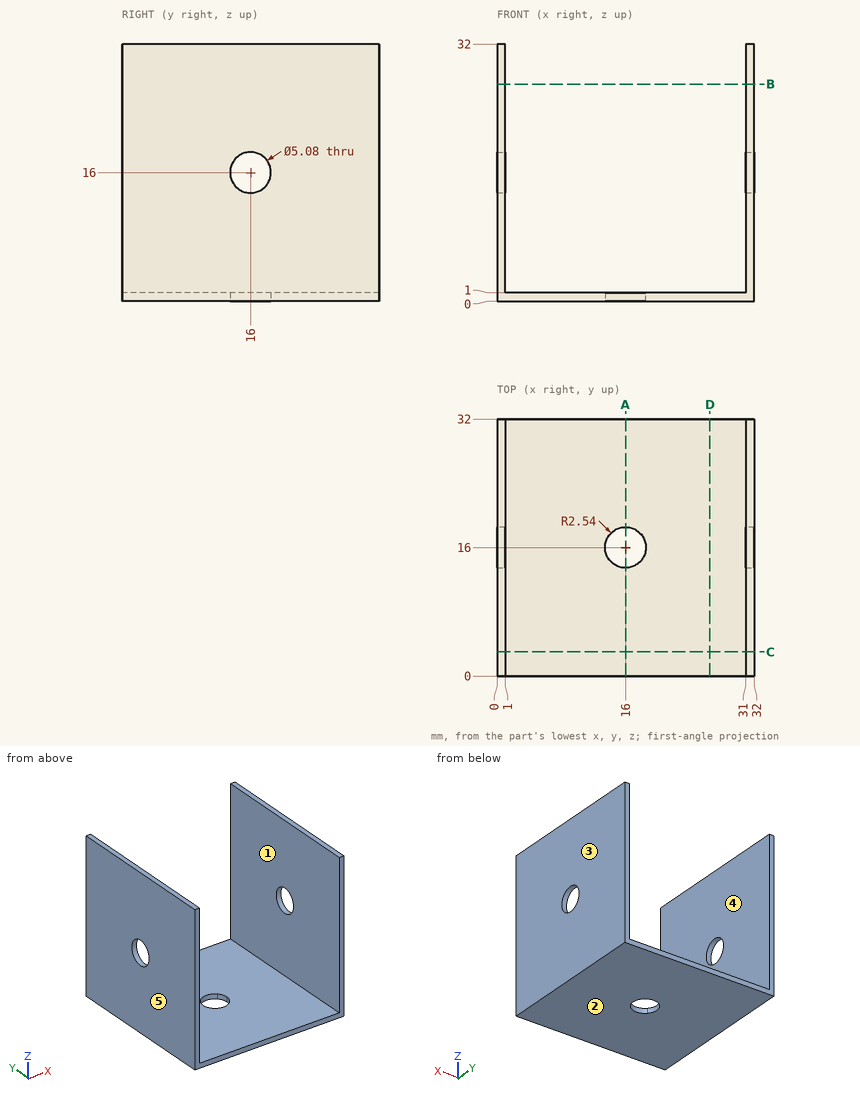
Here's the drawing with two shaded views (mm, measured from the low corner). I have some questions. A direction names the side the tool comes from. Give positions to 0.01 mm unless a question says otherwise; leave off trailing zeros. Loops run counter-clockwise (first coordinate to the right, second up) from the corner with the lowest first, then second, coordinate; pieces in that order, holes last. Notation, with made-up numbers: (-19.5, 84.25) - (-11.5, 84.25) arc R23 ccw to (-11.5, 117.25) - close; hole circle Ø4 at (81, 73). An arc over 180 degrees is marked (long way). Answer in a Markdown table with one row per item. Add a question column.
Q1. If we section it at D-D (x = 26.5): List the corners of the cut face in (y, z) for me.
Q2. For pin 1 (4.5 mm diameter, centred on y = 16, z = 16, fed in from +X); pin 2 (4 mm diameter, centred on x = 25.5, y = 4.5, fed in from +Z), each with a flat end and sliding along its axis, tell me the tip position at first contact or that it passes through.
Q3. We'd pull the mould along X, two halves only. Please class the marked faces 3, 4 and 5: +X half, -X half, draft (parallel to the pull), parting line (faces both ways), or undercut.
Q4. Which directions (+Z, -Z, +X, -X, +Y, -Y) give clear straight access to the entire face, cutting with the end or side of a thin tool? Please do the marked faces 1 and 2.
Q5. If we section it at B-B (z = 27): List the corners of the cut face in (x, y) for me, plus the area to 3 significant figures.
Q6. If we section it at A-A (x = 16): List the corners of the cut face in (y, z) for me.
Q7. If we section it at C-C (y = 3): List the corners of the cut face in (x, z) for me, plus the area to 3 significant figures.
Q8. Please list where these lines run through material, in increasing order: L1, parallel to X at y = 7, z = 19; L2, parallel to Z at x = 0.3, y = 16; L3, parallel to Z at x = 9, y = 9.5. Write a range as from..to.
The answers:
| question | item | result |
|---|---|---|
| 1 | outline | (0, 0) - (32, 0) - (32, 1) - (0, 1) - close |
| 2 | pin 1 | passes through |
| 2 | pin 2 | stops at z = 1 |
| 3 | face 3 | +X half |
| 3 | face 4 | undercut |
| 3 | face 5 | -X half |
| 4 | face 1 | +Z, +Y, -Y |
| 4 | face 2 | -Z, +X, -X, +Y, -Y |
| 5 | outline | (0, 0) - (1, 0) - (1, 32) - (0, 32) - close; (31, 0) - (32, 0) - (32, 32) - (31, 32) - close |
| 5 | area | 64.0 mm^2 |
| 6 | outline | (0, 0) - (13.46, 0) - (13.46, 1) - (0, 1) - close; (18.54, 0) - (32, 0) - (32, 1) - (18.54, 1) - close |
| 7 | outline | (0, 0) - (32, 0) - (32, 32) - (31, 32) - (31, 1) - (1, 1) - (1, 32) - (0, 32) - close |
| 7 | area | 94.0 mm^2 |
| 8 | L1 | x = 0..1, 31..32 |
| 8 | L2 | z = 0..13.46, 18.54..32 |
| 8 | L3 | z = 0..1 |
